Geometry: see drawing. Coordinates: mm, zero at the bounding-box minimum. A direction names the side the tool comes from. Round coordinates to 2 decimals unless told otherwise and drop trailing zeros. Order: outer loops, then holes, each group sorted by start corner. A loop starts at its lowest first (then second) coordinate and runs counter-clockwise, first axis right, second up. Notation, with made-up numbers: (68, 77) - (111, 77) arc R15 ccw to (111, 81) - close; hole circle Ø11 at (51.25, -19). An arc over 180 degrees is marked (long way). Put each result on its own line as item: value. Start each with the question number.
1) Section A-A on y = 96. Output: boundary loops of the cut face in (x, z).
2) Access query for the marked faces 4, 5, 6 and 7. Directions: +Z, -Z, +X, -X, +Y, -Y. A direction counts if a zero-diameter tool reaches every point of the face in a straight line with its end or side. Return the directions, or none.
3) Mould query, pull axis Y, two halves, no side actions, for the marked faces 1, 2 and 3. Classes: +Y half, -Y half, draft (parallel to the pull), parting line (faces both ways), or undercut.
4) Contact query for flat-ended pins moving along their axis: P1, Ø1.5, axis at y = 73.5, z = 76, coming from the -X side; P2, Ø4, axis at y = 89.5, z = 19, coming from the -X side (1 decimal); P3, Ø5, axis at x = 42.5, y = 98.5, coming from the +Z side; P4, Ø1.5, axis at y = 14, z = 35, coming from the -X side (1 decimal). Output: stop coordinate, or through.
5) Section D-D on x = 54. Output: boundary loops of the cut face in (y, z) (1 decimal).
6) Section B-B on x = 34.5. Output: boundary loops of the cut face in (y, z), then the cut area to 3 significant figures.
7) Line query: probe 1 along Y at (x, z) = (53, 73.5); probe 2 along X at (y, z) = (15, 52); probe 3 along X at (y, z) = (28.5, 40). Output: solid intervals per line, ascending. Write a range as [from, to].
8) Section C-C on z = 7. Output: boundary loops of the cut face in (x, y) (1 decimal), then the cut area to 3 significant figures.
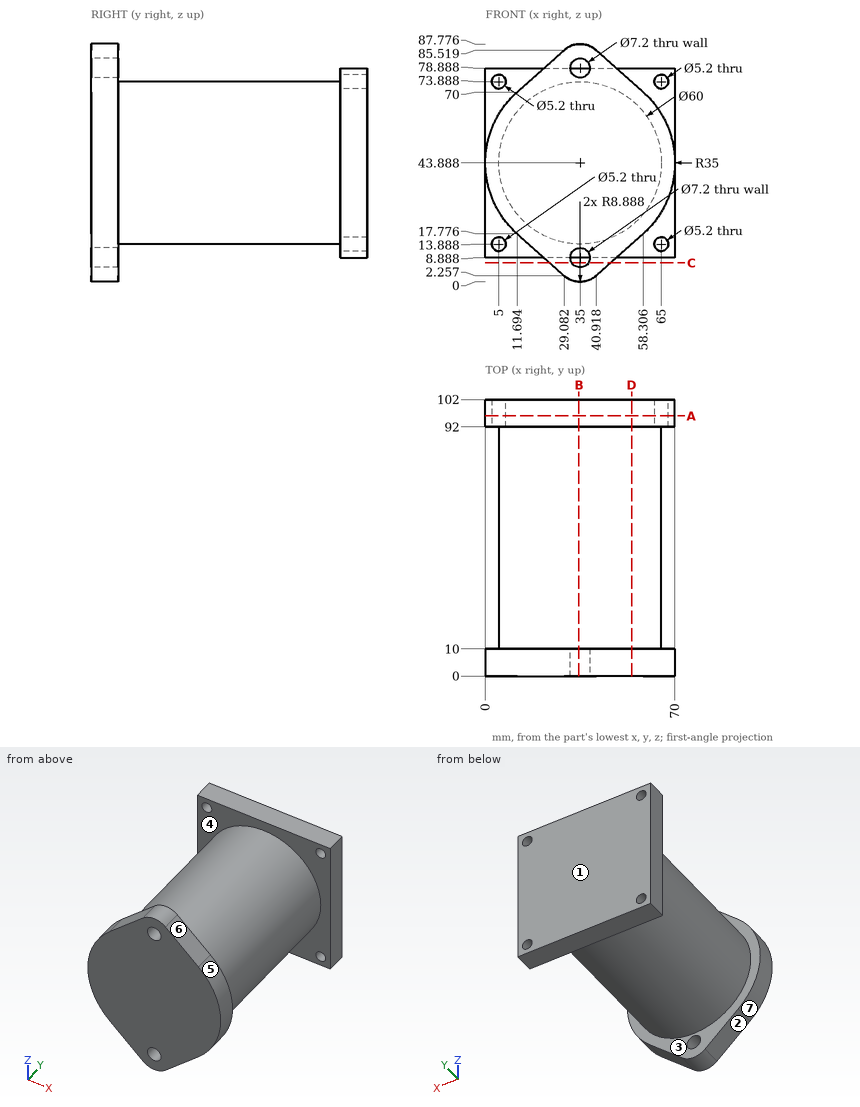
Answer sheet:
1. outline: (0, 8.89) - (70, 8.89) - (70, 78.89) - (0, 78.89) - close; hole circle Ø5.2 at (5, 13.89); hole circle Ø5.2 at (5, 73.89); hole circle Ø5.2 at (65, 13.89); hole circle Ø5.2 at (65, 73.89)
2. face 4: none
2. face 5: +X, -Y
2. face 6: +Z, +X, -Y
2. face 7: -X, -Y
3. face 1: +Y half
3. face 2: draft
3. face 3: undercut
4. P1: through
4. P2: x = 15.6
4. P3: z = 78.89
4. P4: x = 6.1
5. outline: (0, 13.9) - (10, 13.9) - (10, 20.7) - (92, 20.7) - (92, 8.9) - (102, 8.9) - (102, 78.9) - (92, 78.9) - (92, 67.1) - (10, 67.1) - (10, 73.8) - (0, 73.8) - close
6. outline: (0, 0.01) - (10, 0.01) - (10, 5.32) - (0, 5.32) - close; (0, 12.45) - (10, 12.45) - (10, 13.89) - (92, 13.89) - (92, 8.89) - (102, 8.89) - (102, 78.89) - (92, 78.89) - (92, 73.88) - (10, 73.88) - (10, 75.32) - (0, 75.32) - close; (0, 82.45) - (10, 82.45) - (10, 87.76) - (0, 87.76) - close
6. area: 6,350 mm^2
7. probe 1: [0, 10], [92, 102]
7. probe 2: [6.12, 63.88]
7. probe 3: [5.25, 64.75]
8. outline: (23.8, 0) - (31.9, 0) - (31.9, 10) - (23.8, 10) - close; (38.1, 0) - (46.2, 0) - (46.2, 10) - (38.1, 10) - close
8. area: 163 mm^2
